Autodesk Inventor part; units mm, degrees
ref_plane "oben_XY" through (0, 12, 0) normal (0, 1, 0) x (1, 0, 0)
ref_plane "oben_YZ" through (0, 12, 0) normal (1, 0, 0) x (0, 0, -1)
ref_plane "oben_ZX" through (0, 12, 0) normal (0, 0, -1) x (0, 1, 0)
sketch "Sketch_6" plane through (0, 0, 0) normal (0, 0, 1) x (1, 0, 0)
  line L0 (0, 0) -> (0, 16)
  line L1 (0, 16) -> (2.3865, 16)
  line L2 (2.3865, 16) -> (3, 15.3865)
  line L3 (3, 15.3865) -> (3, 12)
  line L4 (3, 12) -> (4.4, 12)
  line L5 (4.4, 12) -> (4.4, 10.5)
  line L6 (4.4, 10.5) -> (12, 10.5)
  line L7 (12, 10.5) -> (12.5, 10)
  line L8 (12.5, 10) -> (12.5, 0.5)
  line L9 (12.5, 0.5) -> (12, 0)
  line L10 (12, 0) -> (0, 0)
  line L11 (0, 0) -> (0, 16)
revolve "Revolution1" add sketch "Sketch_6" angle 360 about axis through (0, 0, 0) along (0, 1, 0)
thread "Thread1"
sketch "Sketch_4" plane through (0, 0, 0) normal (0, 0, 1) x (1, 0, 0)
  line L0 (0, 0) -> (0, 6)
  line L1 (0, 6) -> (2.4585, 6)
  line L2 (2.4585, 6) -> (2.4585, 0.5415)
  line L3 (2.4585, 0.5415) -> (3, 0)
  line L4 (3, 0) -> (0, 0)
  line L5 (0, 0) -> (0, 6)
revolve "Revolution2" cut sketch "Sketch_4" angle 360 about axis through (0, 0, 0) along (0, -1, 0)
thread "Thread2"
sketch "Sketch_5" plane through (0, 0, 0) normal (0, 0, 1) x (1, 0, 0)
  line L0 (0, 10.5) -> (0, 16)
  line L1 (0, 16) -> (2, 16)
  line L2 (2, 16) -> (2, 10.5)
  line L3 (2, 10.5) -> (0, 10.5)
  line L4 (0, 10.5) -> (0, 16)
revolve "Revolution3" cut sketch "Sketch_5" angle 360 about axis through (0, 10.5, 0) along (0, -1, 0)
ref_plane "oben_XY" through (0, 12, 0) normal (0, 1, 0) x (1, 0, 0)
ref_plane "oben_YZ" through (0, 12, 0) normal (1, 0, 0) x (0, 0, -1)
ref_plane "oben_ZX" through (0, 12, 0) normal (0, 0, -1) x (0, 1, 0)
ref_plane "unten_XY" through (0, 0, 0) normal (0, 1, 0) x (1, 0, 0)
ref_plane "unten_YZ" through (0, 0, 0) normal (1, 0, 0) x (0, 0, -1)
ref_plane "unten_ZX" through (0, 0, 0) normal (0, 0, -1) x (0, 1, 0)
properties part number "191203 ESF-4A"
Input: part model. Units: mm. Frame: model coordinates. A direction names the side the tool comes from. Round coordinates to 2 decimals unless told otherwise and drop trailing zeros. Loops run counter-clockwise (first coordinate to the right, second up) from the corner with the lowest first, then second, coordinate; pieces in that order, holes last. Notation, with made-up numbers: (52, -10.75) -> (72, -10.75) arc R14 cw to (72, 12.25) -> close; hole circle Ø7 at (-26, -35.5). An arc over 180 degrees is marked (long way). Use one line per item in the form item = value. Start each with the question number.
Item 1: Mould query, pull axis Z, two halves, no side actions, for faces 4 (the face through (1, 12, 3)), 5 (the face through (4.197, 11.24, 1.322)), 6 (the face through (0, 13, -2)). Classes: pulls with the +Z half, pulls with the -Z half, needs draft (parallel to the pull), parting line crosses it, or undercut.
Item 2: Contact query for flat-ended pins moving along their axis: pin 1 Ø2 at (y, z) = (6.5, -7.5) entering from -X; pin 2 Ø2.5 at (x, z) = (0, 0.5) entering from -Y; pin 3 Ø1.5 at (x, y) = (-2, 14) entering from +Z. Output: stop coordinate, or through.
Item 3: Set-up query: faces 1 (the face through (2.5, 0, 2.5)), 2 (the face through (2.345, 3.233, 0.738)), 3 (the face through (5, 10.5, 0)). Return all of +Z, -Z, +X, -X, +Y, -Y with unobstructed straight access to the full face (end or side cutting, diameter ignored); none if empty.
Item 4: Section query A-A on x = 0. Return the cut outline in (y, z), then the cut area to 3 significant figures.
Item 5: Section query B-B on z = 0. Return the cut outline in (x, y), then the cut area to 3 significant figures.
Item 6: Section query D-D on y = 7.75. Return the cut outline in (x, z).
Item 7: Material intervals for L1, parallel to Z at x = 0, y = 4.7; L2, parallel to Z at x = 0, y = 13.4; L3, parallel to Y at x = 3, z = 6.5, sorted ascending. Write a range as from..to.
Item 8: Section query C-C on y = 1.75. Return the cut outline in (x, z), then the cut area to 3 significant figures.
Ans:
q1.face_4 = needs draft
q1.face_5 = parting line crosses it
q1.face_6 = undercut
q2.pin_1 = -10.68
q2.pin_2 = 6
q2.pin_3 = 2.73
q3.face_1 = +Z, -Z, +X, -X, -Y
q3.face_2 = -Y
q3.face_3 = +Y
q4.outline = (0, -12) -> (0.5, -12.5) -> (10, -12.5) -> (10.5, -12) -> (10.5, -4.4) -> (12, -4.4) -> (12, -3) -> (15.39, -3) -> (16, -2.39) -> (16, -2) -> (10.5, -2) -> (10.5, 2) -> (16, 2) -> (16, 2.39) -> (15.39, 3) -> (12, 3) -> (12, 4.4) -> (10.5, 4.4) -> (10.5, 12) -> (10, 12.5) -> (0.5, 12.5) -> (0, 12) -> (0, 3) -> (0.54, 2.46) -> (6, 2.46) -> (6, -2.46) -> (0.54, -2.46) -> (0, -3) -> close
q4.area = 247 mm^2
q5.outline = (-12.5, 0.5) -> (-12, 0) -> (-3, 0) -> (-2.46, 0.54) -> (-2.46, 6) -> (2.46, 6) -> (2.46, 0.54) -> (3, 0) -> (12, 0) -> (12.5, 0.5) -> (12.5, 10) -> (12, 10.5) -> (4.4, 10.5) -> (4.4, 12) -> (3, 12) -> (3, 15.39) -> (2.39, 16) -> (2, 16) -> (2, 10.5) -> (-2, 10.5) -> (-2, 16) -> (-2.39, 16) -> (-3, 15.39) -> (-3, 12) -> (-4.4, 12) -> (-4.4, 10.5) -> (-12, 10.5) -> (-12.5, 10) -> close
q5.area = 247 mm^2
q6.outline = circle Ø25 at (0, 0)
q7.L1 = -12.5..-2.46, 2.46..12.5
q7.L2 = -3..-2, 2..3
q7.L3 = 0..10.5
q8.outline = circle Ø25 at (0, 0); hole circle Ø4.92 at (0, 0)
q8.area = 472 mm^2
